```python
from build123d import *

# Parameters (mm, degrees)
SKETCH_1_W          = 21.4
SKETCH_1_H          = 8.2
EXTRUDE_1_DEPTH     = 12.1
SKETCH_4_R          = 1.25
CUT_EXTRUDE_3_DEPTH = 8
CUT_EXTRUDE_4_DEPTH = 7.8
SKETCH_7_W          = 1
SKETCH_7_H          = 1
EXTRUDE_2_DEPTH     = 8
CHAMFER_1_SIZE      = 0.15
CHAMFER_2_SIZE      = 0.25
SKETCH_8_W          = 1
SKETCH_8_H          = 1
EXTRUDE_3_DEPTH     = 4
CHAMFER_6_SIZE      = 0.1
CHAMFER_7_SIZE      = 0.2
CHAMFER_10_SIZE     = 0.1
CHAMFER_11_SIZE     = 0.2
CHAMFER_12_SIZE     = 0.1
CHAMFER_13_SIZE     = 0.2
CHAMFER_14_SIZE     = 0.1
CHAMFER_15_SIZE     = 0.2


with BuildPart() as part:
    # Эскиз1 → Бобышка-Вытянуть1 (new body)
    with BuildSketch(Plane.XY):
        Rectangle(SKETCH_1_W, SKETCH_1_H)
    extrude(amount=EXTRUDE_1_DEPTH)

    # Эскиз4 → Вырез-Вытянуть3 (cut)
    with BuildSketch(Plane.XY.offset(12.1)):
        with Locations((-7.5, 0)):
            Circle(SKETCH_4_R)
        with Locations((-2.5, 0)):
            Circle(SKETCH_4_R)
        with Locations((2.5, 0)):
            Circle(SKETCH_4_R)
        with Locations((7.5, 0)):
            Circle(SKETCH_4_R)
    extrude(amount=-CUT_EXTRUDE_3_DEPTH, mode=Mode.SUBTRACT)

    # Эскиз5 → Вырез-Вытянуть4 (cut)
    with BuildSketch(Plane.XY.offset(12.1)):
        with BuildLine():
            Line((-10.245621634, 0), (-10.245621634, 3.292901982))
            Line((-10.245621634, 3.292901982), (0.278509544, 3.292901982))
            Line((0.278509544, 3.292901982), (5.278509544, 3.292901982))
            Line((5.278509544, 3.292901982), (10.278509544, 3.292901982))
            Line((10.278509544, 3.292901982), (10.278509544, -2.548957219))
            Line((10.278509544, -2.548957219), (9.30582632, -2.548957219))
            ThreePointArc((9.30582632, -2.548957219), (7.5, -3.818893996), (5.69417368, -2.548957219))
            Line((5.69417368, -2.548957219), (4.30582632, -2.548957219))
            ThreePointArc((4.30582632, -2.548957219), (2.5, -3.818893996), (0.69417368, -2.548957219))
            Line((0.69417368, -2.548957219), (-0.69417368, -2.548957219))
            ThreePointArc((-0.69417368, -2.548957219), (-2.5, -3.818893996), (-4.30582632, -2.548957219))
            Line((-4.30582632, -2.548957219), (-5.69417368, -2.548957219))
            ThreePointArc((-5.69417368, -2.548957219), (-7.5, -3.818893996), (-9.30582632, -2.548957219))
            Line((-9.30582632, -2.548957219), (-10.245621634, -2.548957219))
            Line((-10.245621634, -2.548957219), (-10.245621634, 0))
        make_face()
    extrude(amount=-CUT_EXTRUDE_4_DEPTH, mode=Mode.SUBTRACT)

    # Эскиз7 → Бобышка-Вытянуть2 (add)
    with BuildSketch(Plane.XY.offset(4.1)):
        with Locations((-2.5, 0)):
            Rectangle(SKETCH_7_W, SKETCH_7_H)
        with Locations((-7.5, 0)):
            Rectangle(SKETCH_7_W, SKETCH_7_H)
        with Locations((2.5, 0)):
            Rectangle(SKETCH_7_W, SKETCH_7_H)
        with Locations((7.5, 0)):
            Rectangle(SKETCH_7_W, SKETCH_7_H)
    extrude(amount=EXTRUDE_2_DEPTH)

    # Фаска1
    chamfer_1_edges = [part.edges().sort_by_distance(p)[0] for p in [
        (-7, -0.5, 8.1),
        (-7, 0.5, 8.1),
        (-8, 0.5, 8.1),
        (-8, -0.5, 8.1),
        (-2, -0.5, 8.1),
        (-2, 0.5, 8.1),
        (-3, 0.5, 8.1),
        (-3, -0.5, 8.1),
    ]]
    chamfer(chamfer_1_edges, length=CHAMFER_1_SIZE)

    # Фаска2
    # the kernel refuses this chamfer: 0.25 mm, written as the material it takes off along each edge
    with BuildSketch(Plane(origin=(-3, -0.992920747, 12.1), x_dir=(-0.02749587661058555, 0, -0.9996219169112968), z_dir=(0, 1, 0)), Plane(origin=(-3.492920747, 0.5, 12.1), x_dir=(0, 0.027495876610586414, -0.9996219169112968), z_dir=(1, 0, 0)), Plane(origin=(-2, 0.992920747, 12.1), x_dir=(0.027495876610586414, 0, -0.9996219169112968), z_dir=(0, -1, 0)), Plane(origin=(-1.507079253, -0.5, 12.1), x_dir=(0, -0.027495876610586414, -0.9996219169112968), z_dir=(-1, 0, 0)), Plane(origin=(-7, 0.992920747, 12.1), x_dir=(0.02749587661058555, 0, -0.9996219169112968), z_dir=(0, -1, 0)), Plane(origin=(-6.507079253, -0.5, 12.1), x_dir=(0, -0.027495876610586414, -0.9996219169112968), z_dir=(-1, 0, 0)), Plane(origin=(-8, -0.992920747, 12.1), x_dir=(-0.027495876610589005, 0, -0.9996219169112968), z_dir=(0, 1, 0)), Plane(origin=(-8.492920747, 0.5, 12.1), x_dir=(0, 0.027495876610586414, -0.9996219169112968), z_dir=(1, 0, 0))) as chamfer_2_piece_1:
        Polygon((CHAMFER_2_SIZE * 0.999621916911, -CHAMFER_2_SIZE * 0.0274958766106), (-CHAMFER_2_SIZE * 0.0274958766106, -CHAMFER_2_SIZE * 0.999621916911), (0, 0), align=None)
    extrude(amount=1.985841494, mode=Mode.SUBTRACT)

    # Эскиз8 → Бобышка-Вытянуть3 (add)
    with BuildSketch(Plane(origin=(0, -4.1, 0), x_dir=(-1, 0, 0), z_dir=(0, 0, 1))):
        with Locations((2.5, -3.75)):
            Rectangle(SKETCH_8_W, SKETCH_8_H)
        with Locations((7.5, -3.75)):
            Rectangle(SKETCH_8_W, SKETCH_8_H)
        with Locations((-2.5, -3.75)):
            Rectangle(SKETCH_8_W, SKETCH_8_H)
        with Locations((-7.5, -3.75)):
            Rectangle(SKETCH_8_W, SKETCH_8_H)
    extrude(amount=-EXTRUDE_3_DEPTH)

    # Фаска6
    chamfer_6_edges = [part.edges().sort_by_distance(p)[0] for p in [
        (3, -0.5, 8.1),
        (3, 0.5, 8.1),
        (2, 0.5, 8.1),
        (2, -0.5, 8.1),
    ]]
    chamfer(chamfer_6_edges, length=CHAMFER_6_SIZE)

    # Фаска7
    # the kernel refuses this chamfer: 0.2 mm, written as the material it takes off along each edge
    with BuildSketch(Plane(origin=(3, 0.914336598, 12.1), x_dir=(0.02749587661058742, 0, -0.9996219169112966), z_dir=(0, -1, 0)), Plane(origin=(3.414336598, -0.5, 12.1), x_dir=(0, -0.02749587661058634, -0.9996219169112966), z_dir=(-1, 0, 0)), Plane(origin=(2, -0.914336598, 12.1), x_dir=(-0.02749587661058634, 0, -0.9996219169112966), z_dir=(0, 1, 0)), Plane(origin=(1.585663402, 0.5, 12.1), x_dir=(0, 0.02749587661058634, -0.9996219169112966), z_dir=(1, 0, 0))) as chamfer_7_piece_1:
        Polygon((CHAMFER_7_SIZE * 0.999621916911, -CHAMFER_7_SIZE * 0.0274958766106), (-CHAMFER_7_SIZE * 0.0274958766106, -CHAMFER_7_SIZE * 0.999621916911), (0, 0), align=None)
    extrude(amount=1.828673195, mode=Mode.SUBTRACT)

    # Фаска10
    chamfer_10_edges = [part.edges().sort_by_distance(p)[0] for p in [
        (-7, 0.15, -2),
        (-7, -0.85, -2),
        (-8, -0.85, -2),
        (-8, 0.15, -2),
        (-2, 0.15, -2),
        (-2, -0.85, -2),
        (-3, -0.85, -2),
        (-3, 0.15, -2),
        (3, 0.15, -2),
        (3, -0.85, -2),
        (2, -0.85, -2),
        (2, 0.15, -2),
    ]]
    chamfer(chamfer_10_edges, length=CHAMFER_10_SIZE)

    # Фаска11
    # the kernel refuses this chamfer: 0.2 mm, written as the material it takes off along each edge
    with BuildSketch(Plane(origin=(-7, 0.564336598, -4), x_dir=(0.027495876610587302, 0, 0.9996219169112966), z_dir=(0, -1, 0)), Plane(origin=(-8.414336598, 0.15, -4), x_dir=(0, 0.027495876610586355, 0.9996219169112966), z_dir=(1, 0, 0)), Plane(origin=(-8, -1.264336598, -4), x_dir=(-0.027495876610587302, 0, 0.9996219169112966), z_dir=(0, 1, 0)), Plane(origin=(-6.585663402, -0.85, -4), x_dir=(0, -0.027495876610586223, 0.9996219169112966), z_dir=(-1, 0, 0)), Plane(origin=(-1.585663402, -0.85, -4), x_dir=(0, -0.027495876610586223, 0.9996219169112966), z_dir=(-1, 0, 0)), Plane(origin=(-3, -1.264336598, -4), x_dir=(-0.027495876610587302, 0, 0.9996219169112966), z_dir=(0, 1, 0)), Plane(origin=(-3.414336598, 0.15, -4), x_dir=(0, 0.027495876610586355, 0.9996219169112966), z_dir=(1, 0, 0)), Plane(origin=(-2, 0.564336598, -4), x_dir=(0.027495876610586223, 0, 0.9996219169112966), z_dir=(0, -1, 0)), Plane(origin=(2, -1.264336598, -4), x_dir=(-0.027495876610586223, 0, 0.9996219169112966), z_dir=(0, 1, 0)), Plane(origin=(1.585663402, 0.15, -4), x_dir=(0, 0.027495876610586355, 0.9996219169112966), z_dir=(1, 0, 0)), Plane(origin=(3, 0.564336598, -4), x_dir=(0.027495876610587302, 0, 0.9996219169112966), z_dir=(0, -1, 0)), Plane(origin=(3.414336598, -0.85, -4), x_dir=(0, -0.027495876610586223, 0.9996219169112966), z_dir=(-1, 0, 0))) as chamfer_11_piece_1:
        Polygon((CHAMFER_11_SIZE * 0.999621916911, CHAMFER_11_SIZE * 0.0274958766106), (-CHAMFER_11_SIZE * 0.0274958766106, CHAMFER_11_SIZE * 0.999621916911), (0, 0), align=None)
    extrude(amount=1.828673195, mode=Mode.SUBTRACT)

    # Фаска12
    chamfer_12_edges = [part.edges().sort_by_distance(p)[0] for p in [
        (8, 0.15, -2),
        (8, -0.85, -2),
        (7, -0.85, -2),
        (7, 0.15, -2),
    ]]
    chamfer(chamfer_12_edges, length=CHAMFER_12_SIZE)

    # Фаска13
    # the kernel refuses this chamfer: 0.2 mm, written as the material it takes off along each edge
    with BuildSketch(Plane(origin=(6.585663402, 0.15, -4), x_dir=(0, 0.027495876610586355, 0.9996219169112966), z_dir=(1, 0, 0)), Plane(origin=(8, 0.564336598, -4), x_dir=(0.027495876610587302, 0, 0.9996219169112966), z_dir=(0, -1, 0)), Plane(origin=(7, -1.264336598, -4), x_dir=(-0.027495876610587302, 0, 0.9996219169112966), z_dir=(0, 1, 0)), Plane(origin=(8.414336598, -0.85, -4), x_dir=(0, -0.027495876610586223, 0.9996219169112966), z_dir=(-1, 0, 0))) as chamfer_13_piece_1:
        Polygon((CHAMFER_13_SIZE * 0.999621916911, CHAMFER_13_SIZE * 0.0274958766106), (-CHAMFER_13_SIZE * 0.0274958766106, CHAMFER_13_SIZE * 0.999621916911), (0, 0), align=None)
    extrude(amount=1.828673195, mode=Mode.SUBTRACT)

    # Фаска14
    chamfer_14_edges = [part.edges().sort_by_distance(p)[0] for p in [
        (8, -0.5, 8.1),
        (8, 0.5, 8.1),
        (7, 0.5, 8.1),
        (7, -0.5, 8.1),
    ]]
    chamfer(chamfer_14_edges, length=CHAMFER_14_SIZE)

    # Фаска15
    # the kernel refuses this chamfer: 0.2 mm, written as the material it takes off along each edge
    with BuildSketch(Plane(origin=(7, -0.914336598, 12.1), x_dir=(-0.02749587661058742, 0, -0.9996219169112966), z_dir=(0, 1, 0)), Plane(origin=(8.414336598, -0.5, 12.1), x_dir=(0, -0.02749587661058634, -0.9996219169112966), z_dir=(-1, 0, 0)), Plane(origin=(8, 0.914336598, 12.1), x_dir=(0.02749587661058742, 0, -0.9996219169112966), z_dir=(0, -1, 0)), Plane(origin=(6.585663402, 0.5, 12.1), x_dir=(0, 0.02749587661058634, -0.9996219169112966), z_dir=(1, 0, 0))) as chamfer_15_piece_1:
        Polygon((CHAMFER_15_SIZE * 0.999621916911, -CHAMFER_15_SIZE * 0.0274958766106), (-CHAMFER_15_SIZE * 0.0274958766106, -CHAMFER_15_SIZE * 0.999621916911), (0, 0), align=None)
    extrude(amount=1.828673195, mode=Mode.SUBTRACT)


solid = part.part
```
Source: CAD feature listing. Evaluate the final solid. Frame: model axes, mm. A direction names the side the tool comes from. Give positions to 0.01 mm unless a question says otherwise; leave off trailing zeros. Loops run counter-clockwise (first coordinate to the right, second up) from the corner with the lowest first, then second, coordinate; pieces in that order, holes last. Notation, with made-up numbers: (57.5, -20.75) - (80.5, -20.75) arc R17 cw to (80.5, -10.75) - close; hole circle Ø11 at (40.5, 50.25). An arc over 180 degrees is marked (long way). Use CSV: the item, a comma, the result in double quotes. Start each with the question number.
1. Section D-D (x = 7.5). Output: boundary loops of the cut face in (y, z).
2. Section A-A (y = 2.75). Output: boundary loops of the cut face in (x, z), then the cut area to 3 significant figures.
3. Section B-B (x = -7.5). Output: boundary loops of the cut face in (y, z), then the cut area to 3 significant figures.
4. Section C-C (z = 8.5). Count the separate pieces of the cut face and the enclosed holes in it, then the cut area to 3 significant figures.
5. Reachability of faces 1 (the flat face through (10.7, 0, 6)), 2 (the flat face through (-7.5, -0.85, -1.9)), 3 (the flat face through (10, -2.549, 8)) from +Z, -Z, +X, -X, +Y, -Y: full face, straight path, thin tool, end or side. Return the list, or none.
6. Pin query (flat end, axial travel): pin 1 (1.2 mm diameter, centred on x = 8, y = -0.5, fed in from +Z); pin 2 (0.6 mm diameter, centred on y = -0.5, z = -2.5, fed in from +X); pin 3 (0.6 mm diameter, centred on y = -0.5, z = -1, fed in from -X); pin 4 (0.9 mm diameter, centred on x = -2.5, z = -2, fed in from -Y). Return the tip coordinate at first contact, or that it passes through.
7. Draft query along Y for faces 4 (the cylindrical face through (2.53, -3.82, 8.25)), 5 (the flat face through (0, -4.1, 6)), 6 (the flat face through (0, 0, 0)). Return one class per face: +Y half, -Y half, draft (parallel to the pull), parting line (faces both ways), or undercut.
8. Ray query, L1, parallel to Y at x = -2.5, z = 4.2; L2, parallel to X at y = 0, z = 4.35; L3, parallel to Y at x = -5.5, z = 5.75. Return the intervals inside material, ascending.
Response:
1,outline,"(-4.1, 0) - (-0.85, 0) - (-0.85, -3.8) - (-0.65, -4) - (-0.05, -4) - (0.15, -3.8) - (0.15, 0) - (4.1, 0) - (4.1, 12.1) - (3.29, 12.1) - (3.29, 4.3) - (1.25, 4.3) - (1.25, 4.1) - (0.5, 4.1) - (0.5, 11.9) - (0.3, 12.1) - (-0.3, 12.1) - (-0.5, 11.9) - (-0.5, 4.1) - (-1.25, 4.1) - (-1.25, 4.3) - (-3.82, 4.3) - (-3.82, 12.1) - (-4.1, 12.1) - close"
2,outline,"(-10.7, 0) - (10.7, 0) - (10.7, 12.1) - (10.28, 12.1) - (10.28, 4.3) - (-10.25, 4.3) - (-10.25, 12.1) - (-10.7, 12.1) - close"
2,area,"98.9 mm²"
3,outline,"(-4.1, 0) - (-0.85, 0) - (-0.85, -3.8) - (-0.65, -4) - (-0.05, -4) - (0.15, -3.8) - (0.15, 0) - (4.1, 0) - (4.1, 12.1) - (3.29, 12.1) - (3.29, 4.3) - (1.25, 4.3) - (1.25, 4.1) - (0.5, 4.1) - (0.5, 11.85) - (0.25, 12.1) - (-0.25, 12.1) - (-0.5, 11.85) - (-0.5, 4.1) - (-1.25, 4.1) - (-1.25, 4.3) - (-3.82, 4.3) - (-3.82, 12.1) - (-4.1, 12.1) - close"
3,area,"55.1 mm²"
4,separate pieces,"5"
4,enclosed holes,"1"
4,area,"46.1 mm²"
5,face 1,"+Z, -Z, +X, +Y, -Y"
5,face 2,"-Z, +X, -X, -Y"
5,face 3,"+Z"
6,pin 1,"z = 12.1"
6,pin 2,"x = 8"
6,pin 3,"x = -8"
6,pin 4,"y = -0.85"
7,face 4,"undercut"
7,face 5,"-Y half"
7,face 6,"draft"
8,L1,"-4.1 to -1.25, -0.5 to 0.5, 1.25 to 4.1"
8,L2,"-10.7 to -10.25, -8 to -7, -3 to -2, 2 to 3, 7 to 8, 10.28 to 10.7"
8,L3,"-4.1 to -2.55, 3.29 to 4.1"
